Could you check a few things on this model? Use its own coordinates, in mm. Round coordinates to 2 decimals unless told otherwise and drop trailing zeros. Order: outer loops, then holes, each group sorted by start corner. A loop starts at its lowest first (then second) coordinate and runs counter-clockwise, first axis right, second up.
```python
from build123d import *

# Parameters (mm, degrees)
F1_DEPTH = 10
F2_R     = 2
F3_DEPTH = 25


with BuildPart() as f1:
    # F0 (on Front) → F1 (new body)
    with BuildSketch(Plane.XZ):
        with BuildLine():
            Line((7.211103, 12), (4, 12))
            Line((4, 12), (4, -12))
            Line((4, -12), (7.211103, -12))
            ThreePointArc((7.211103, -12), (9.899495, -9.899495), (12, -7.211103))
            Line((12, -7.211103), (12, 7.211103))
            ThreePointArc((12, 7.211103), (9.899495, 9.899495), (7.211103, 12))
        make_face()
    extrude(amount=-F1_DEPTH)

    # F2 (on face) → F3 (cut)
    with BuildSketch(Plane(origin=(4, 0, 0), x_dir=(0, -1, 0), z_dir=(-1, 0, 0))):
        with Locations((-5, 0)):
            Circle(F2_R)
    extrude(amount=-F3_DEPTH, mode=Mode.SUBTRACT)


solid = f1.part
```
Q1. Imagine slicing it at D-D, the plane y = 7.25. Please give me the cut outline in (x, z), then the cut area to 3 significant figures.
Q2. Imagine slicing it at B-B, the plane y = 5. Please give me the cut outline in (x, z).
Q3. I need wall thicknesses on L1, parallel to Z at x = 8.75, y = 5.25; L2, parallel to Z at x = 9.75, y = 5; L3, parallel to Z at x = 11, y = 8. Which ranges of each line are inside material? Lowest first, please.
Q4. Imagine slicing it at C-C, the plane x = 6.25. Please give me the cut outline in (y, z).
Q5. For P1, Ø3, axis at y = 5, z = 0, coming from the -X side, with a flat end and sliding along its axis, tell me the tip position at first contact or that it passes through.
Q6. Imagine slicing it at A-A, the plane z = 0. Please give me the cut outline in (x, y), then the cut area to 3 significant figures.
Filled in:
1. outline: (4, -12) - (7.21, -12) arc R14 ccw to (12, -7.21) - (12, 7.21) arc R14 ccw to (7.21, 12) - (4, 12) - close
1. area: 173 mm2
2. outline: (4, -12) - (7.21, -12) arc R14 ccw to (12, -7.21) - (12, -2) - (4, -2) - close; (4, 2) - (12, 2) - (12, 7.21) arc R14 ccw to (7.21, 12) - (4, 12) - close
3. L1: z = -10.93 to -1.98, 1.98 to 10.93
3. L2: z = -10.05 to -2, 2 to 10.05
3. L3: z = -8.66 to 8.66
4. outline: (0, -12) - (10, -12) - (10, 12) - (0, 12) - close; hole circle Ø4 at (5, 0)
5. P1: passes through
6. outline: (4, 0) - (12, 0) - (12, 3) - (4, 3) - close; (4, 7) - (12, 7) - (12, 10) - (4, 10) - close
6. area: 48.0 mm2
